Read the model definition and answer for the solid it produces. Units are mm, in the model's axes. A direction names the side the tool comes from. Coordinates: 2 decimals unless noted, no trailing zeros. Write each loop counter-clockwise with the first axis right and the second up, starting at its lowest first coordinate (ties: lowest second). Pieces come first, ordered by that corner, then holes.
(1) Given pin 1 (2 mm diameter, centred on x = -1.5, z = 123, fed in from -Y); pin 2 (6 mm diameter, centred on x = 5, z = 18, fed in from -Y); pin 3 (5 mm diameter, centred on x = 0, z = 134, fed in from -Y), each flat-ended and moving along its own axis, determine where each tip first touches the part or whether it passes through.
(2) Section A-A on y = 0 is taken. Write down the section's boundary in (x, z), then the cut area to 3 significant figures.
(3) Which of the six approach directions +Z, -Z, +X, -X, +Y, -Y give full straight-line access (tool end or side, diameter ignored) to faces 1 (the flat face through (0, 0, 165.608)), 2 (the cylindrical face through (-1.34, 10.2, 109.73))?
(4) Section C-C on z = 17.5 is taken. Write down the section's boundary in (x, y).
(5) Section B-B on x = 0.5 is taken. Write down the section's boundary in (y, z), then the cut area to 3 significant figures.
(6) Find the intervals of material crossed by probe 1 along Z at (x, y) = (-3.25, 8); probe 2 along Z at (x, y) = (-9.25, 1); probe 3 along Y at (x, z) = (4.5, 114.5), in increasing order.
from build123d import *

# Parameters (mm, degrees)
F0_R     = 12.954
F0_R_2   = 11.43
F1_DEPTH = 45.974
F0_R_3   = 10.287
F2_DEPTH = 92.202
F0_R_4   = 9.271
F3_DEPTH = 127.762
F0_R_5   = 7.62
F4_DEPTH = 147.574
F5_DEPTH = 165.608


with BuildPart() as f1:
    # F0 (on Top) → F1 (new body)
    with BuildSketch(Plane.XY):
        Circle(F0_R)
        Circle(F0_R_2, mode=Mode.SUBTRACT)
    extrude(amount=F1_DEPTH)

    # F0 (on Top) → F2 (join)
    with BuildSketch(Plane.XY):
        Circle(F0_R_2)
        Circle(F0_R_3, mode=Mode.SUBTRACT)
    extrude(amount=F2_DEPTH)

    # F0 (on Top) → F3 (join)
    with BuildSketch(Plane.XY):
        Circle(F0_R_3)
        Circle(F0_R_4, mode=Mode.SUBTRACT)
    extrude(amount=F3_DEPTH)

    # F0 (on Top) → F4 (join)
    with BuildSketch(Plane.XY):
        Circle(F0_R_4)
        Circle(F0_R_5, mode=Mode.SUBTRACT)
    extrude(amount=F4_DEPTH)

    # F0 (on Top) → F5 (join)
    with BuildSketch(Plane.XY):
        Circle(F0_R_5)
    extrude(amount=F5_DEPTH)


solid = f1.part
Response:
1. pin 1: stops at y = -10.27
1. pin 2: stops at y = -12.8
1. pin 3: stops at y = -9.27
2. outline: (-12.95, 0) - (12.95, 0) - (12.95, 45.97) - (11.43, 45.97) - (11.43, 92.2) - (10.29, 92.2) - (10.29, 127.76) - (9.27, 127.76) - (9.27, 147.57) - (7.62, 147.57) - (7.62, 165.61) - (-7.62, 165.61) - (-7.62, 147.57) - (-9.27, 147.57) - (-9.27, 127.76) - (-10.29, 127.76) - (-10.29, 92.2) - (-11.43, 92.2) - (-11.43, 45.97) - (-12.95, 45.97) - close
2. area: 3,620 mm2
3. face 1: +Z, +X, -X, +Y, -Y
3. face 2: +Z
4. outline: circle Ø25.91 at (0, 0)
5. outline: (-12.94, 0) - (12.94, 0) - (12.94, 45.97) - (11.42, 45.97) - (11.42, 92.2) - (10.27, 92.2) - (10.27, 127.76) - (9.26, 127.76) - (9.26, 147.57) - (7.6, 147.57) - (7.6, 165.61) - (-7.6, 165.61) - (-7.6, 147.57) - (-9.26, 147.57) - (-9.26, 127.76) - (-10.27, 127.76) - (-10.27, 92.2) - (-11.42, 92.2) - (-11.42, 45.97) - (-12.94, 45.97) - close
5. area: 3,620 mm2
6. probe 1: z = 0 to 147.57
6. probe 2: z = 0 to 127.76
6. probe 3: y = -9.25 to 9.25
